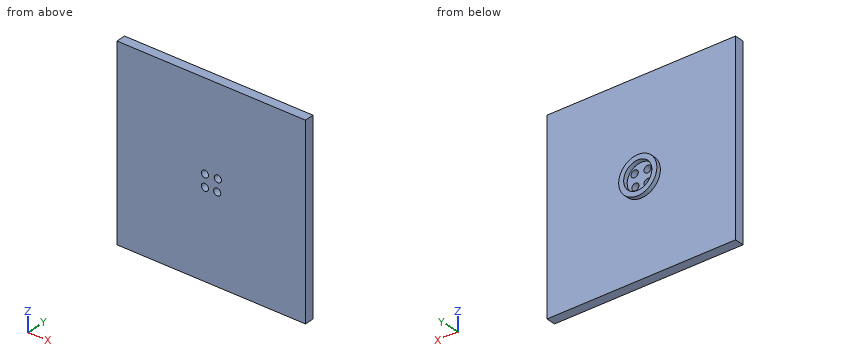
Autodesk Inventor part; units mm, degrees
ref_plane "YZ Plane" through (0, 0, 0) normal (1, 0, 0) x (0, 1, 0)
ref_plane "XZ Plane" through (0, 0, 0) normal (0, 1, 0) x (-1, 0, 0)
ref_plane "XY Plane" through (0, 0, 0) normal (0, 0, 1) x (1, 0, 0)
sketch "Sketch1" plane through (0, 0, 0) normal (0, 1, 0) x (-1, 0, 0)
  line L0 (0, 0) -> (-127, 0)
  line L1 (-127, 0) -> (-127, -127)
  line L2 (-127, -127) -> (0, -127)
  line L3 (0, -127) -> (0, 0)
  dimension "d0" = 127
  dimension "d1" = 127
extrude "Extrusion1" add sketch "Sketch1" along normal blind 6.35
sketch "Sketch2" plane through (0, 6.35, 0) normal (0, 1, 0) x (1, 0, 0)
  line L0 (0, 0) -> (127, 0)
  line L1 (127, 0) -> (127, 127)
  line L2 (56.7828, 56.7828) -> (70.2172, 70.2172)
  line L3 (127, 127) -> (127, 0)
  line L4 (70.2172, 56.7828) -> (56.7828, 70.2172)
  line L5 (0, 127) -> (0, 0)
  circle A0 centre (63.5, 63.5) radius 9.4996
  circle A1 centre (63.5, 63.5) radius 12.8477
extrude "Extrusion2" add sketch "Sketch2" along normal blind 2.9972
sketch "Sketch3" plane through (63.5, 6.35, -63.5) normal (0, 1, 0) x (1, 0, 0)
  circle A0 centre (0, 0) radius 9.4996
  line L0 (9.4891, 0.446) -> (9.7729, 0.446) construction
  line L1 (-5.8104, 5.9947) -> (-6.6345, 6.7989)
  circle A1 centre (3.7745, 4.4415) radius 2.413
  circle A2 centre (4.4123, -3.9814) radius 2.413
  circle A3 centre (-4.3831, -3.9179) radius 2.413
  circle A4 centre (-4.0835, 4.3094) radius 2.413
  line L2 (6.1393, -5.6667) -> (6.9589, -6.4665)
  line L3 (5.4598, 6.1684) -> (6.3421, 7.0725)
  line L4 (-6.9155, -6.5129) -> (-6.0684, -5.6448)
  line L5 (6.9589, -6.4665) -> (6.1393, -5.6667)
  point P0 (-63.5, -63.5)
hole "Hole1" at (67.4966, 6.35, -67.8963) direction (0, -1, 0) diameter 4.826 end through all
hole "Hole2" at (59.2369, 6.35, -68.1627) direction (0, -1, 0) diameter 4.826 end through all
hole "Hole3" at (59.2369, 6.35, -59.903) direction (0, -1, 0) diameter 4.826 end through all
hole "Hole4" at (67.9123, 6.35, -59.5186) direction (0, -1, 0) diameter 4.826 end through all
Work out the finished part from the listing and answer in its coordinate system (mm). Give positions to 0.01 mm unless a question says otherwise; leave off trailing zeros. Loops run counter-clockwise (first coordinate to the right, second up) from the corner with the lowest first, then second, coordinate; pieces in that order, holes last. Notation, with made-up numbers: (54, -19) -> (74, -19) arc R11 ccw to (74, -13) -> close; hole circle Ø10 at (48, 26.5). An arc over 180 degrees is marked (long way). Use a Markdown table: item, result. Add a question column.
1) The part is cut by section C-C, the plane x = 23.5. Determine the outline of the cut face in (y, z).
2) Consider line 1 along X through (y, z) = (0.5, -68); line 2 along Z through (x, y) = (66, 4.25); line 3 along Y through (x, z) = (29, -20.5). Determine where each line is inside the solid, lowest interval first.
3) The part is cut by section B-B, the plane z = -98.5. Determine the outline of the cut face in (x, y), plus the area to 3 significant figures.
4) The part is cut by section A-A, the plane x = 63.5. Determine the outline of the cut face in (y, z), plus the area to 3 significant figures.
5) Each of these flat-tipped pins is pushed along its axis until it touches: P1, Ø3, axis at x = 67.5, z = -67.9, coming from the +Y side; P2, Ø5.5, axis at x = 59.24, z = -68.16, coming from the +Y side. Where does it stop, or does it pass through?
Reported:
| question | item | result |
|---|---|---|
| 1 | outline | (0, -127) -> (6.35, -127) -> (6.35, 0) -> (0, 0) -> close |
| 2 | line 1 | x = 0 to 56.83, 61.64 to 65.09, 69.91 to 127 |
| 2 | line 2 | z = -127 to -69.79, -66 to -60.99, -58.05 to 0 |
| 2 | line 3 | y = 0 to 6.35 |
| 3 | outline | (0, 0) -> (127, 0) -> (127, 6.35) -> (0, 6.35) -> close |
| 3 | area | 806 mm^2 |
| 4 | outline | (0, -127) -> (6.35, -127) -> (6.35, -76.35) -> (9.35, -76.35) -> (9.35, -73) -> (6.35, -73) -> (6.35, -54) -> (9.35, -54) -> (9.35, -50.65) -> (6.35, -50.65) -> (6.35, 0) -> (0, 0) -> close |
| 4 | area | 827 mm^2 |
| 5 | P1 | passes through |
| 5 | P2 | stops at y = 6.35 |
